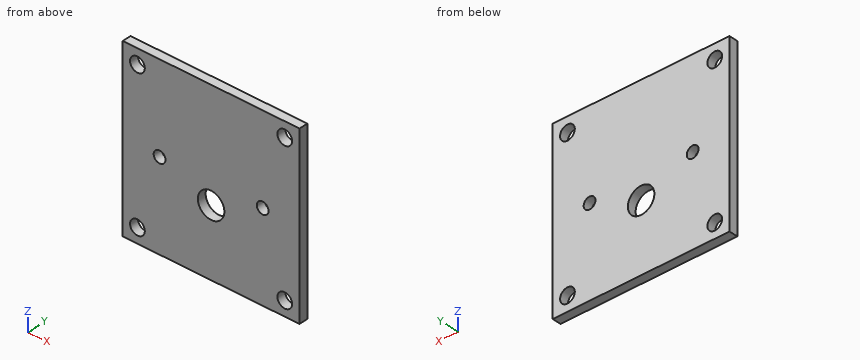
from build123d import *

# Parameters (mm, degrees)
SKETCH1_W           = 60
SKETCH1_H           = 60
SKETCH1_R           = 2.5
SKETCH1_R_2         = 4.5
SKETCH1_R_3         = 2
BOSS_EXTRUDE1_DEPTH = 3


with BuildPart() as part:
    # Sketch1 → Boss-Extrude1 (new body)
    with BuildSketch(Plane(origin=(0, 0, 0), x_dir=(1, 0, 0), z_dir=(0, 1, 0))):
        Rectangle(SKETCH1_W, SKETCH1_H)
        with Locations((-25, -25)):
            Circle(SKETCH1_R, mode=Mode.SUBTRACT)
        with Locations((25, -25)):
            Circle(SKETCH1_R, mode=Mode.SUBTRACT)
        with BuildLine():
            Line((-13.555441712, -3.5), (-17.495441712, -3.5))
            ThreePointArc((-17.495441712, -3.5), (-20.995441712, 0), (-17.495441712, 3.5))
            Line((-17.495441712, 3.5), (-13.555441712, 3.5))
            ThreePointArc((-13.555441712, 3.5), (0, 14), (13.555441712, 3.5))
            Line((13.555441712, 3.5), (17.495441712, 3.5))
            ThreePointArc((17.495441712, 3.5), (20.995441712, 0), (17.495441712, -3.5))
            Line((17.495441712, -3.5), (13.555441712, -3.5))
            ThreePointArc((13.555441712, -3.5), (0, -14), (-13.555441712, -3.5))
        make_face(mode=Mode.SUBTRACT)
        with Locations((-25, 25)):
            Circle(SKETCH1_R, mode=Mode.SUBTRACT)
        with Locations((25, 25)):
            Circle(SKETCH1_R, mode=Mode.SUBTRACT)
        with BuildLine():
            ThreePointArc((-13.999088699, -0.159736057), (-13.878125858, -1.843264133), (-13.555441712, -3.5))
            ThreePointArc((-13.555441712, -3.5), (0, -14), (13.555441712, -3.5))
            ThreePointArc((13.555441712, -3.5), (13.878125858, -1.843264133), (13.999088699, -0.159736057))
            ThreePointArc((13.999088699, -0.159736057), (13.995441712, 0), (13.999088699, 0.159736057))
            ThreePointArc((13.999088699, 0.159736057), (13.878125858, 1.843264133), (13.555441712, 3.5))
            ThreePointArc((13.555441712, 3.5), (0, 14), (-13.555441712, 3.5))
            ThreePointArc((-13.555441712, 3.5), (-13.878125858, 1.843264133), (-13.999088699, 0.159736057))
            ThreePointArc((-13.999088699, 0.159736057), (-13.995441712, 0), (-13.999088699, -0.159736057))
        make_face()
        with Locations((0, 7)):
            Circle(SKETCH1_R_2, mode=Mode.SUBTRACT)
        with BuildLine():
            ThreePointArc((-17.495441712, 3.5), (-20.995441712, 0), (-17.495441712, -3.5))
            Line((-17.495441712, -3.5), (-13.555441712, -3.5))
            ThreePointArc((-13.555441712, -3.5), (-13.878125858, -1.843264133), (-13.999088699, -0.159736057))
            ThreePointArc((-13.999088699, -0.159736057), (-14, 0), (-13.999088699, 0.159736057))
            ThreePointArc((-13.999088699, 0.159736057), (-13.878125858, 1.843264133), (-13.555441712, 3.5))
            Line((-13.555441712, 3.5), (-17.495441712, 3.5))
        make_face()
        with Locations((-17.495441712, 0)):
            Circle(SKETCH1_R_3, mode=Mode.SUBTRACT)
        with BuildLine():
            ThreePointArc((13.999088699, -0.159736057), (13.878125858, -1.843264133), (13.555441712, -3.5))
            Line((13.555441712, -3.5), (17.495441712, -3.5))
            ThreePointArc((17.495441712, -3.5), (20.995441712, 0), (17.495441712, 3.5))
            Line((17.495441712, 3.5), (13.555441712, 3.5))
            ThreePointArc((13.555441712, 3.5), (13.878125858, 1.843264133), (13.999088699, 0.159736057))
            ThreePointArc((13.999088699, 0.159736057), (13.999772173, 0.079869328), (14, 0))
            ThreePointArc((14, 0), (13.999772173, -0.079869328), (13.999088699, -0.159736057))
        make_face()
        with Locations((17.495441712, 0)):
            Circle(SKETCH1_R_3, mode=Mode.SUBTRACT)
    extrude(amount=BOSS_EXTRUDE1_DEPTH)


solid = part.part
Work out the finished part from the listing and answer in its coordinate system (mm). Give positions to 0.01 mm unless a question says otherwise; leave off trailing zeros. Write each loop counter-clockwise with the first axis right and the second up, starting at its lowest first coordinate (ties: lowest second). Pieces come first, ordered by that corner, then holes. Notation, with made-up numbers: M -5.75,28.5 L 27.25,28.5 A25 cw 27.25,60.5 Z; hole C 41.25,28.5 d8. An arc over 180 degrees is marked long. Answer as CSV lines item,"result".
Q1. A cutting plane is placed at B-B on x = -17.5. Write down the section's boundary in (y, z).
A:
outline,"M 0,-30 L 3,-30 L 3,-2 L 0,-2 Z; M 0,2 L 3,2 L 3,30 L 0,30 Z"
Q2. A cutting plane is placed at D-D on x = -25. Write down the section's boundary in (y, z).
A:
outline,"M 0,-30 L 3,-30 L 3,-27.5 L 0,-27.5 Z; M 0,-22.5 L 3,-22.5 L 3,22.5 L 0,22.5 Z; M 0,27.5 L 3,27.5 L 3,30 L 0,30 Z"
Q3. A cutting plane is placed at C-C on y = 2.4. Count the separate pieces of the cut face and the enclosed holes in it, plus the area to 3 significant figures.
A:
separate pieces,"1"
enclosed holes,"9"
area,"3,430 mm²"
Q4. Find the intervals of material crossed by probe 1 along Z at (x, y) = (-25, 1.1); probe 2 along Z at (x, y) = (24, 2.6); probe 3 along X at (y, z) = (0.4, -0.5), in increasing order. Write a range as [from, to].
A:
probe 1,"z = [-30, -27.5], [-22.5, 22.5], [27.5, 30]"
probe 2,"z = [-30, -27.29], [-22.71, 22.71], [27.29, 30]"
probe 3,"x = [-30, -19.43], [-15.56, 15.56], [19.43, 30]"
Q5. A cutting plane is placed at A-A on z = -7. Write down the section's boundary in (x, y).
A:
outline,"M -30,0 L -4.5,0 L -4.5,3 L -30,3 Z; M 4.5,0 L 30,0 L 30,3 L 4.5,3 Z"
